from build123d import *

# Parameters (mm, degrees)
ESQUISSE2_W          = 30.5
ESQUISSE2_H          = 8.25
BASE_EXTRUSION_DEPTH = 31.5
ESQUISSE3_W          = 30.5
ESQUISSE3_H          = 15.5
BOSS_EXTRU_2_DEPTH   = 2.8
ESQUISSE4_R          = 2.65
BOSS_EXTRU_3_DEPTH   = 12


with BuildPart() as part:
    # Esquisse2 → Base-Extrusion (new body)
    with BuildSketch(Plane.XY):
        with Locations((-45.33773679, 19.692248255)):
            Rectangle(ESQUISSE2_W, ESQUISSE2_H)
    extrude(amount=BASE_EXTRUSION_DEPTH)

    # Esquisse3 → Boss.-Extru.2 (add)
    with BuildSketch(Plane.XY.offset(31.5)):
        with Locations((-45.33773679, 23.317248255)):
            Rectangle(ESQUISSE3_W, ESQUISSE3_H)
    extrude(amount=-BOSS_EXTRU_2_DEPTH)

    # Esquisse4 → Boss.-Extru.3 (add)
    with BuildSketch(Plane.ZY.offset(60.58773679)):
        with Locations(Location((8.1, 18.217248255, 0), (0, 0, 270))):
            Circle(ESQUISSE4_R)
    boss_extru_3 = extrude(amount=BOSS_EXTRU_3_DEPTH)

    # Symétrie1: Boss.-Extru.3 across plane
    add(boss_extru_3.mirror(Plane.ZY.offset(45.33773679)))


solid = part.part
Here's how the part is built. I have some questions about the finished solid (model axes, mm). A direction names the side the tool comes from. Round coordinates to 2 decimals unless told otherwise and drop trailing zeros. Order: outer loops, then holes, each group sorted by start corner. A loop starts at its lowest first (then second) coordinate and runs counter-clockwise, first axis right, second up. Notation, with made-up numbers: (39.25, -9.5) -> (54.25, -9.5) arc R17 cw to (54.25, 13.5) -> close; hole circle Ø6 at (-7, 73.25). An arc over 180 degrees is marked (long way). Return JSON: item names as keys, results as strings.
Q1. Which directions (+Z, -Z, +X, -X, +Y, -Y) give clear straight access to the entire face, cutting with the end or side of a thin tool? Please do faces 4 (the flat face through (-46, 15.567, 16)), 5 (the flat face through (-46, 23.817, 14)), 6 (the cylindrical face through (-24.172, 20.865, 8.217)).
Filled sheet:
{"face 4": "+Z, -Z, +X, -X, -Y", "face 5": "-Z, +X, -X, +Y", "face 6": "+X"}
Q2. I need wall thicknesses on line 1 along X through (y, z) = (17.5, 22.5); line 2 along Y through (x, z) = (-36, 6.5); line 3 along Z through (x, y) = (-56, 25.5). Which ranges of each line are inside material? Lowest first, please. Write a range as from..to.
Filled sheet:
{"line 1": "x = -60.59..-30.09", "line 2": "y = 15.57..23.82", "line 3": "z = 28.7..31.5"}
Q3. If we section it at C-C on y = 28.25: List the corners of the cut face in (x, z) for me, plus the area to 3 significant figures.
Filled sheet:
{"outline": "(-60.59, 28.7) -> (-30.09, 28.7) -> (-30.09, 31.5) -> (-60.59, 31.5) -> close", "area": "85.4 mm^2"}
Q4. If we section it at A-A on x = -26: List the corners of the cut face in (y, z) for me, plus the area to 3 significant figures.
Filled sheet:
{"outline": "circle Ø5.3 at (18.22, 8.1)", "area": "22.1 mm^2"}
Q5. If we section it at B-B on z = 9.5: List the corners of the cut face in (x, y) for me, plus the area to 3 significant figures.
Filled sheet:
{"outline": "(-72.59, 15.97) -> (-60.59, 15.97) -> (-60.59, 15.57) -> (-30.09, 15.57) -> (-30.09, 15.97) -> (-18.09, 15.97) -> (-18.09, 20.47) -> (-30.09, 20.47) -> (-30.09, 23.82) -> (-60.59, 23.82) -> (-60.59, 20.47) -> (-72.59, 20.47) -> close", "area": "360 mm^2"}
Q6. If we mould it in two halves opening along X, with no side actions, what happens to faces 1 (the cylindrical face through (-66.504, 20.865, 8.217)), 2 (the flat face through (-30.088, 20, 16)), 3 (the flat face through (-72.588, 18, 8))? For each: released by +X, released by -X, zero draft, split by the parting line, or undercut.
Filled sheet:
{"face 1": "zero draft", "face 2": "released by +X", "face 3": "released by -X"}
Q7. If we section it at D-D on x = -33: List the corners of the cut face in (y, z) for me, plus the area to 3 significant figures.
Filled sheet:
{"outline": "(15.57, 0) -> (23.82, 0) -> (23.82, 28.7) -> (31.07, 28.7) -> (31.07, 31.5) -> (15.57, 31.5) -> close", "area": "280 mm^2"}
Q8. For pin 1 Ø4 at (x, z) = (-26.5, 10.5) entering from +Y; pin 2 Ø3.5 at (x, y) = (-38, 27) entering from -Z; pin 3 Ø14.5 at (x, z) = (-49.5, 16) entering from +Y; pin 4 Ø4 at (x, y) = (-43.5, 25.5) entering from -Z, each with a flat end and sliding along its axis, tell me the tip position at first contact or that it passes through.
Filled sheet:
{"pin 1": "stops at y = 20.84", "pin 2": "stops at z = 28.7", "pin 3": "stops at y = 23.82", "pin 4": "stops at z = 0"}
